Design review of the part built by this model. Coordinates are the model's own, in mm. Face numbers are marked on the shaded views. A direction names the side the tool comes from. Give positions to 0.01 mm unless a question says otherwise; leave off trailing zeros. Order: outer loops, then holes, each group sorted by start corner. A loop starts at its lowest first (then second) coordinate and runs counter-clockwise, first axis right, second up. Notation, with made-up numbers: (-38, 47.5) - (-21, 47.5) arc R23 ccw to (-21, 63.5) - close; hole circle Ø10 at (-37, -21). An arc over 180 degrees is marked (long way). Write each question's results on one line, items separated by ' | '. Start each with the question number.
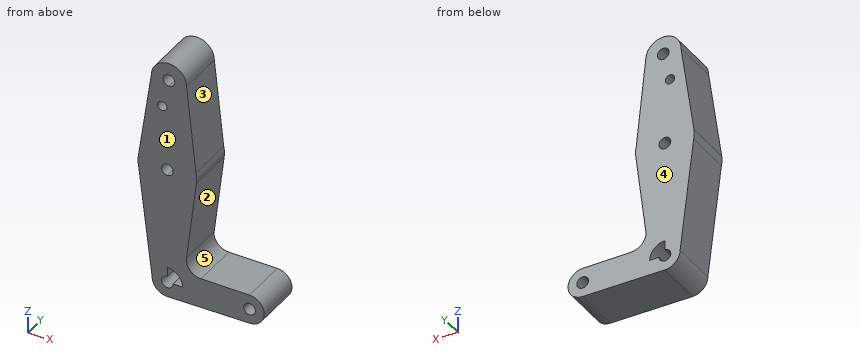
```python
from build123d import *

# Parameters (mm, degrees)
F0_R     = 2.4970860884
F1_DEPTH = 25.4


with BuildPart() as f1:
    # F0 (on Front) → F1 (new body)
    with BuildSketch(Plane.XZ):
        with BuildLine():
            ThreePointArc((-34.058996731, 41.8151793819), (-34.0587916512, 41.8512656744), (-34.058723291, 41.8873524848))
            ThreePointArc((-34.058723291, 41.8873524848), (-43.6204916456, 51.412281518), (-53.108439425, 41.8138163235))
            ThreePointArc((-53.108439425, 41.8138163235), (-50.3500442403, 35.1834337942), (-43.7455028396, 32.3637264748))
            ThreePointArc((-43.7455028396, 32.3637264748), (-36.931754808, 35.0699526651), (-34.058996731, 41.8151793819))
        make_face()
        with BuildLine():
            ThreePointArc((-40.408723291, 41.8873524848), (-41.3578068156, 39.6233028289), (-43.6376498072, 38.7128104815))
            ThreePointArc((-43.6376498072, 38.7128104815), (-45.8096397664, 44.1514021407), (-40.408723291, 41.8873524848))
        make_face(mode=Mode.SUBTRACT)
        with BuildLine():
            ThreePointArc((-43.7455028396, 32.3637264748), (-50.3500442403, 35.1834337942), (-53.108439425, 41.8138163235))
            Line((-53.108439425, 41.8138163235), (-60.1423228458, -6.5331159404))
            ThreePointArc((-60.1423228458, -6.5331159404), (-54.6939631735, 3.2120648216), (-44.1770394505, 6.9600625014))
            Line((-44.1770394505, 6.9600625014), (-43.7455028396, 32.3637264748))
        make_face()
        with Locations((-47.1983999014, 26.2127500027)):
            Circle(F0_R, mode=Mode.SUBTRACT)
        with BuildLine():
            Line((-28.9755803483, -5.3544250476), (-34.058996731, 41.8151793819))
            ThreePointArc((-34.058996731, 41.8151793819), (-36.931754808, 35.0699526651), (-43.7455028396, 32.3637264748))
            Line((-43.7455028396, 32.3637264748), (-44.1770394505, 6.9600625014))
            ThreePointArc((-44.1770394505, 6.9600625014), (-34.4539621393, 3.4227233349), (-28.9755803483, -5.3544250476))
        make_face()
        with BuildLine():
            Line((-60.1696796465, -6.7211510996), (-60.1423228458, -6.5331159404))
            ThreePointArc((-60.1423228458, -6.5331159404), (-60.156282583, -6.6270925889), (-60.1696796465, -6.7211510996))
        make_face()
        with BuildLine():
            ThreePointArc((-44.1770394505, 6.9600625014), (-54.6939631735, 3.2120648216), (-60.1423228458, -6.5331159404))
            Line((-60.1423228458, -6.5331159404), (-60.1696796465, -6.7211510996))
            ThreePointArc((-60.1696796465, -6.7211510996), (-60.3127983863, -9.4433635349), (-59.9880891038, -12.149927297))
            ThreePointArc((-59.9880891038, -12.149927297), (-54.4622551015, -21.2294539506), (-44.4466720315, -24.7876475152))
            Line((-44.4466720315, -24.7876475152), (-44.4466720315, -12.0876475152))
            ThreePointArc((-44.4466720315, -12.0876475152), (-47.6215575303, -8.8856832847), (-44.3927455153, -5.7381055119))
            Line((-44.3927455153, -5.7381055119), (-44.1770394505, 6.9600625014))
        make_face()
        with BuildLine():
            ThreePointArc((-28.5716720315, -8.9126475152), (-28.6729723153, -7.1221106504), (-28.9755803483, -5.3544250476))
            ThreePointArc((-28.9755803483, -5.3544250476), (-34.4539621393, 3.4227233349), (-44.1770394505, 6.9600625014))
            Line((-44.1770394505, 6.9600625014), (-44.3927455153, -5.7381055119))
            ThreePointArc((-44.3927455153, -5.7381055119), (-42.1826223756, -6.6867310398), (-41.2716720315, -8.9126475152))
            ThreePointArc((-41.2716720315, -8.9126475152), (-42.2016080012, -11.1577115455), (-44.4466720315, -12.0876475152))
            Line((-44.4466720315, -12.0876475152), (-44.4466720315, -24.7876475152))
            ThreePointArc((-44.4466720315, -24.7876475152), (-34.115422457, -20.9659004882), (-28.7584623121, -11.3407539379))
            Line((-28.7584623121, -11.3407539379), (-28.6355797608, -10.3356676158))
            ThreePointArc((-28.6355797608, -10.3356676158), (-28.5876570117, -9.6248747269), (-28.5716720315, -8.9126475152))
        make_face()
        with BuildLine():
            ThreePointArc((-44.4466720315, -24.7876475152), (-54.4622551015, -21.2294539506), (-59.9880891038, -12.149927297))
            Line((-59.9880891038, -12.149927297), (-52.6740726434, -72.4126475152))
            ThreePointArc((-52.6740726434, -72.4126475152), (-50.2643227957, -66.594996751), (-44.4466720315, -64.1852469033))
            Line((-44.4466720315, -64.1852469033), (-44.4466720315, -24.7876475152))
        make_face()
        with BuildLine():
            ThreePointArc((-28.7584623121, -11.3407539379), (-28.68900545, -10.839190768), (-28.6355797608, -10.3356676158))
            Line((-28.6355797608, -10.3356676158), (-28.7584623121, -11.3407539379))
        make_face()
        with BuildLine():
            ThreePointArc((-28.7584623121, -11.3407539379), (-34.115422457, -20.9659004882), (-44.4466720315, -24.7876475152))
            Line((-44.4466720315, -24.7876475152), (-44.4466720315, -64.1852469033))
            ThreePointArc((-44.4466720315, -64.1852469033), (-38.6456689688, -66.5783965525), (-36.2194057783, -72.3656280761))
            Line((-36.2194057783, -72.3656280761), (-7.9373703756, -72.2039941384))
            ThreePointArc((-7.9373703756, -72.2039941384), (-5.6286753497, -66.5620325034), (0, -64.2211314758))
            Line((0, -64.2211314758), (-26.2460871779, -64.1999413714))
            ThreePointArc((-26.2460871779, -64.1999413714), (-32.1947833248, -61.5168387322), (-34.1311079114, -55.2849311015))
            Line((-34.1311079114, -55.2849311015), (-28.7584623121, -11.3407539379))
        make_face()
        with BuildLine():
            ThreePointArc((-44.4466720315, -64.1852469033), (-50.2643227957, -66.594996751), (-52.6740726434, -72.4126475152))
            ThreePointArc((-52.6740726434, -72.4126475152), (-50.2643227957, -78.2302982795), (-44.4466720315, -80.6400481271))
            Line((-44.4466720315, -80.6400481271), (-44.2453363669, -80.6375842797))
            ThreePointArc((-44.2453363669, -80.6375842797), (-38.5582685977, -78.1586744756), (-36.2192714196, -72.4126475152))
            ThreePointArc((-36.2192714196, -72.4126475152), (-36.2193050093, -72.3891376997), (-36.2194057783, -72.3656280761))
            Line((-36.2194057783, -72.3656280761), (-41.2717238813, -72.3945024502))
            ThreePointArc((-41.2717238813, -72.3945024502), (-41.271684994, -72.4035749457), (-41.2716720315, -72.4126475152))
            ThreePointArc((-41.2716720315, -72.4126475152), (-46.6917360618, -74.6577115455), (-44.4466720315, -69.2376475152))
            Line((-44.4466720315, -69.2376475152), (-44.4466720315, -64.1852469033))
        make_face()
        with BuildLine():
            Line((-44.2453363669, -80.6375842797), (-44.4466720315, -80.6400481271))
            ThreePointArc((-44.4466720315, -80.6400481271), (-44.3459966616, -80.6394321422), (-44.2453363669, -80.6375842797))
        make_face()
        with BuildLine():
            Line((-7.9373703756, -72.2039941384), (-36.2194057783, -72.3656280761))
            ThreePointArc((-36.2194057783, -72.3656280761), (-36.2193050093, -72.3891376997), (-36.2192714196, -72.4126475152))
            ThreePointArc((-36.2192714196, -72.4126475152), (-38.5582685977, -78.1586744756), (-44.2453363669, -80.6375842797))
            Line((-44.2453363669, -80.6375842797), (0, -80.0961314758))
            ThreePointArc((0, -80.0961314758), (-5.5965989724, -77.7873068255), (-7.9373703756, -72.2039941384))
        make_face()
        with BuildLine():
            ThreePointArc((0, -64.2211314758), (-5.6286753497, -66.5620325034), (-7.9373703756, -72.2039941384))
            ThreePointArc((-7.9373703756, -72.2039941384), (-5.5965989724, -77.7873068255), (0, -80.0961314758))
            ThreePointArc((0, -80.0961314758), (5.6126600757, -77.7712915515), (7.9375, -72.1586314758))
            ThreePointArc((7.9375, -72.1586314758), (5.6126600757, -66.5459714001), (0, -64.2211314758))
        make_face()
        with BuildLine():
            ThreePointArc((3.175, -72.1586314758), (0.0090725696, -75.3336185133), (-3.1749481502, -72.1767765408))
            ThreePointArc((-3.1749481502, -72.1767765408), (-0.0090725696, -68.9836444383), (3.175, -72.1586314758))
        make_face(mode=Mode.SUBTRACT)
    extrude(amount=F1_DEPTH)


solid = f1.part
```
Q1. Machinability: for the marked faces 1 and 2, which of the approach directions +Z, -Z, +X, -X, +Y, -Y give a long, thin tool a straight path to every point of the face, cutting with its end or side? Answer none if there is none.
Q2. For line 1 (Z direction, x = -46, y = -18.75); line 2 (Z direction, x = -1, y = -23); line 3 (Z direction, x = 2, y = -10), list the stretches that pass through material, from the lowest coordinate up. Write a range as [from, to].
Q3. Add section C-C (z = 0). Give the boundary of the cut face in (x, y), plus the area to 3 significant figures.
Q4. Draft analysis for pull direction Z (two halves, no side actions). For the marked faces 3, 4 and 5, state which applies: pulls with the +Z half, pulls with the -Z half, needs draft (parallel to the pull), parting line crosses it, or undercut.
Q5. Add section B-B (x = -24). Give the boundary of the cut face in (y, z).
Q6. Insertion check: pin 1 Ø1.5 at (x, z) = (-31, -52) entering from -Y; pin 2 Ø1.5 at (y, z) = (-13, -19) entering from +X; pin 3 Ø6 at (y, z) = (-7, 3.5) entering from -X; pin 4 Ø1.5 at (x, y) = (-3.5, -3.5) entering from +Z. Each pin has a flat end and moves straight along its axis. Give the tip position at first contact, or say it passes through.
Q7. Add section A-A (y = -2.75). Give the number of separate pieces and of enclosed holes in the cut face, plus the area to 3 significant figures.
Verdict:
1) face 1: +Z, -Z, +X, -X, -Y | face 2: +X, +Y, -Y
2) line 1: z = [-80.49, -75.18], [-69.64, -11.68], [-6.14, 24.02], [28.4, 39.83], [43.95, 51.1] | line 2: z = [-80.11, -75.17], [-69.15, -64.22] | line 3: z = [-79.84, -74.62], [-69.69, -64.48]
3) outline: (-59.19, -25.4) - (-29.55, -25.4) - (-29.55, 0) - (-59.19, 0) - close | area: 753 mm2
4) face 3: pulls with the +Z half | face 4: needs draft | face 5: undercut
5) outline: (-25.4, -80.39) - (0, -80.39) - (0, -64.2) - (-25.4, -64.2) - close
6) pin 1: passes through | pin 2: stops at x = -29.6 | pin 3: stops at x = -59.12 | pin 4: stops at z = -64.22
7) separate pieces: 1 | enclosed holes: 5 | area: 3,600 mm2
